```python
from build123d import *

# Parameters (mm, degrees)
BODYS_R       = 3
BODY_DEPTH    = 15
FLATS_W       = 10
FLATS_H       = 6
FLAT_DEPTH    = 0.5
GROOVES_W     = 0.75
GROOVES_H     = 0.7
CHAMFER1_SIZE = 0.5


with BuildPart() as part:
    # BodyS → Body (new, symmetric)
    with BuildSketch(Plane(origin=(0, 0, 0), x_dir=(0, 0, -1), z_dir=(1, 0, 0))):
        Circle(BODYS_R)
    extrude(amount=BODY_DEPTH, both=True)

    # FlatS → Flat (cut)
    with BuildSketch(Plane(origin=(0, 3, 0), x_dir=(1, 0, 0), z_dir=(0, 1, 0))):
        with Locations((10, 0)):
            Rectangle(FLATS_W, FLATS_H)
    extrude(amount=-FLAT_DEPTH, mode=Mode.SUBTRACT)

    # GrooveS → Groove for ANSI B27.7 - 3AM1-6, Basic External Retaining Ring1 (revolve, cut)
    with BuildSketch(Plane(origin=(-15, 0, 0), x_dir=(0, 0, -1), z_dir=(0, -1, 0))):
        with Locations((3.225, 16.85)):
            Rectangle(GROOVES_W, GROOVES_H)
    revolve(axis=Axis((-62.5, 0, 0), (1, 0, 0)), mode=Mode.SUBTRACT)

    # Chamfer1
    chamfer1_edges = [part.edges().sort_by_distance(p)[0] for p in [
        (15, -2.643382037, 1.418637165),
    ]]
    chamfer(chamfer1_edges, length=CHAMFER1_SIZE - 0.0001)  # a hair under: the kernel refuses the full size


solid = part.part
```
The listing builds one solid part. Answer for the finished solid, in the listing's coordinates (mm). A direction names the side the tool comes from. Coordinates: 2 decimals unless noted, no trailing zeros. Write each loop counter-clockwise with the first axis right and the second up, starting at its lowest first coordinate (ties: lowest second). Pieces come first, ordered by that corner, then holes. Notation, with made-up numbers: (19.5, 85.5) - (58.5, 85.5) arc R31 ccw to (58.5, 110.5) - close; hole circle Ø10 at (44.5, 89.5). An arc over 180 degrees is marked (long way). One line per item, written item: value.
1) Each of these flat-tipped pins is pushed along its axis until it touches: pin 1 Ø3 at (x, y) = (-11.5, 0.5) entering from -Z; pin 2 Ø2 at (x, z) = (10, -1) entering from +Y; pin 3 Ø0.6 at (y, z) = (3, 0.5) entering from +X; pin 4 Ø1 at (x, y) = (0.5, -1.5) entering from +Z. Where does it stop, or does it pass through?
Geometry check:
pin 1: stops at z = -3
pin 2: stops at y = 2.5
pin 3: stops at x = 5
pin 4: stops at z = 2.83
2) Consider line 1 along Y through (x, z) = (-2.5, -0.2); line 2 along Z through (x, y) = (-8.75, 0.9); line 3 along Y through (x, z) = (-1.25, -1.15). Determine where each line is inside the solid, lowest interval first. Write a range as from..to.
Geometry check:
line 1: y = -2.99..2.99
line 2: z = -2.86..2.86
line 3: y = -2.77..2.77
3) For a pull along X with two mould halves and no side action, classify faces 3 (the flat face through (-15, 0, 0)), 4 (the cylindrical face through (1.855, -1.734, 2.262)), 5 (the flat face through (15, 0, 0)) as pulls with the +X half, pulls with the -X half, needs draft (parallel to the pull), parting line crosses it, or undercut.
Geometry check:
face 3: pulls with the -X half
face 4: undercut
face 5: pulls with the +X half
4) A tool of negligible diameter and unlimited length cuts with its end or side. For faces 1 (the flat face through (10, 2.5, 0)), 2 (the cylindrical face through (8.44, -2.93, 0.65)), from which of +Z, -Z, +X, -X, +Y, -Y can it reach the whole face along a straight path? Write none if from no direction.
Geometry check:
face 1: +Z, -Z, +X, +Y
face 2: +X, -X
5) Find section A-A (x = -11.25). Give the vertices of the cut face in (y, z).
Geometry check:
outline: circle Ø6 at (0, 0)
